from build123d import *

# Parameters (mm, degrees)
SKETCH_1_R          = 22.5
SKETCH_1_R_2        = 1.65
EXTRUDE_1_DEPTH     = 4
SKETCH_2_R          = 12.5
SKETCH_2_R_2        = 8
EXTRUDE_2_DEPTH     = 10
SKETCH_3_R          = 4
CUT_EXTRUDE_1_DEPTH = 3
SKETCH_4_R          = 8
EXTRUDE_3_DEPTH     = 2
SKETCH_3_3_R        = 1.6
CUT_EXTRUDE_2_DEPTH = 10
CHAMFER_1_SIZE      = 2
CHAMFER_1_SIZE2     = 3.464101615


with BuildPart() as part:
    # Sketch 1 → Extrude 1 (new body)
    with BuildSketch(Plane(origin=(0, 0, 0), x_dir=(1, 0, 0), z_dir=(0, 1, 0))):
        with Locations(Location((0, 0, 0), (0, 0, 270))):
            Circle(SKETCH_1_R)
        with Locations(Location((-18, 0, 0), (0, 0, 270))):
            Circle(SKETCH_1_R_2, mode=Mode.SUBTRACT)
        with Locations(Location((18, 0, 0), (0, 0, 270))):
            Circle(SKETCH_1_R_2, mode=Mode.SUBTRACT)
        with Locations(Location((0, 18, 0), (0, 0, 270))):
            Circle(SKETCH_1_R_2, mode=Mode.SUBTRACT)
        with Locations(Location((0, -18, 0), (0, 0, 270))):
            Circle(SKETCH_1_R_2, mode=Mode.SUBTRACT)
    extrude(amount=EXTRUDE_1_DEPTH)

    # Sketch 2 → Extrude 2 (add)
    with BuildSketch(Plane(origin=(0, 4, 0), x_dir=(1, 0, 0), z_dir=(0, 1, 0))):
        with Locations(Location((0, 0, 0), (0, 0, 270))):
            Circle(SKETCH_2_R)
        with Locations(Location((0, 0, 0), (0, 0, 270))):
            Circle(SKETCH_2_R_2, mode=Mode.SUBTRACT)
    extrude(amount=EXTRUDE_2_DEPTH)

    # Sketch 3 → Cut-Extrude 1 (cut)
    with BuildSketch(Plane.XZ):
        with Locations(Location((0, 0, 0), (0, 0, 270))):
            Circle(SKETCH_3_R)
    extrude(amount=-CUT_EXTRUDE_1_DEPTH, mode=Mode.SUBTRACT)

    # Sketch 4 → Extrude 3 (add)
    with BuildSketch(Plane(origin=(0, 4, 0), x_dir=(1, 0, 0), z_dir=(0, 1, 0))):
        with Locations(Location((0, 0, 0), (0, 0, 270))):
            Circle(SKETCH_4_R)
    extrude(amount=EXTRUDE_3_DEPTH)

    # Sketch 3_3 → Cut-Extrude 2 (cut)
    with BuildSketch(Plane.XZ):
        with Locations(Location((0, 0, 0), (0, 0, 270))):
            Circle(SKETCH_3_3_R)
    extrude(amount=-CUT_EXTRUDE_2_DEPTH, mode=Mode.SUBTRACT)

    # Chamfer 1
    chamfer_1_edges = [part.edges().sort_by_distance(p)[0] for p in [
        (0, 4, -12.5),
    ]]
    chamfer_1_side = [part.faces().sort_by_distance(p)[0] for p in [
        (0, 4, -21.863603897),
    ]]
    chamfer(chamfer_1_edges, length=CHAMFER_1_SIZE, length2=CHAMFER_1_SIZE2, reference=chamfer_1_side[0])


solid = part.part
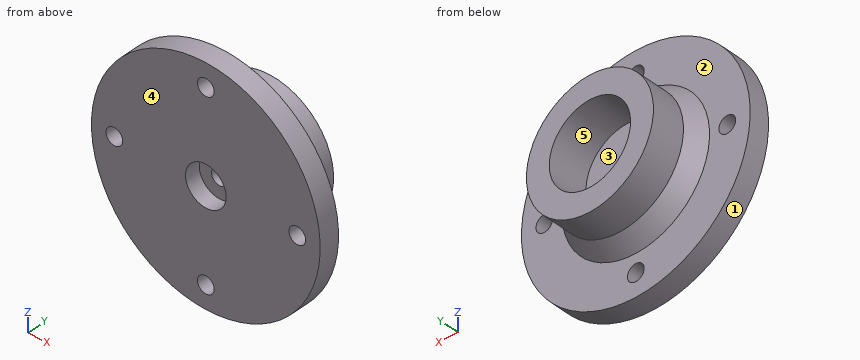
Geometry: final body of the model. Coordinates: model frame, mm. Face numbers are marked on the shaded views. A direction names the side the tool comes from. Round coordinates to 2 decimals unless told otherwise and drop trailing zeros. Loops run counter-clockwise (first coordinate to the right, second up) from the corner with the lowest first, then second, coordinate; pieces in that order, holes last. Notation, with made-up numbers: (84.5, -35) - (100.5, -35) arc R22 cw to (100.5, 4) - close; hole circle Ø9 at (4, 14.25). An arc over 180 degrees is marked (long way). Write each question's results on one line, items separated by ' | '. Start each with the question number.
1) Mould query, pull axis X, two halves, no side actions, for the marked faces 1, 2 and 3. Classes: released by +X, released by -X, zero draft, split by the parting line, or undercut.
2) Access query for the marked faces 4 and 5. Directions: +Z, -Z, +X, -X, +Y, -Y. A direction counts if a zero-diameter tool reaches every point of the face in a straight line with its end or side. Return the directions, or none.
3) Cut plane A-A on x = 18. Return loops of the section in (y, z), then the cut area to 3 significant figures.
4) Line query: probe 1 along X at (y, z) = (0.95, 0); probe 2 along X at (y, z) = (3.05, 0); probe 3 along X at (y, z) = (12, 0). Output: solid intervals per line, ascending. Write a range as [from, to].
5) Cut plane B-B on z = 0. Count the separate pieces of the cut face and the enclosed holes in it, then the cut area to 3 significant figures.
6) Cut plane D-D on z = 18. Return loops of the section in (x, y).
7) First-contact query: P1, Ø5, axis at x = 0, z = 0, coming from the -Y side; P2, Ø5, axis at y = 10.5, z = -10, coming from the +X side; P3, Ø8, axis at y = 6.5, z = 3.5, coming from the +X side. Flat tips, straight axial feed; report the tip coordinate or a pass-through.
Verdict:
1) face 1: split by the parting line | face 2: zero draft | face 3: undercut
2) face 4: +Z, -Z, +X, -X, -Y | face 5: +Y
3) outline: (0, -13.5) - (4, -13.5) - (4, -1.65) - (0, -1.65) - close; (0, 1.65) - (4, 1.65) - (4, 13.5) - (0, 13.5) - close | area: 94.8 mm2
4) probe 1: x = [-22.5, -19.65], [-16.35, -4], [4, 16.35], [19.65, 22.5] | probe 2: x = [-22.5, -19.65], [-16.35, -1.6], [1.6, 16.35], [19.65, 22.5] | probe 3: x = [-12.5, -8], [8, 12.5]
5) separate pieces: 4 | enclosed holes: 0 | area: 249 mm2
6) outline: (-13.5, 0) - (-1.65, 0) - (-1.65, 4) - (-13.5, 4) - close; (1.65, 0) - (13.5, 0) - (13.5, 4) - (1.65, 4) - close
7) P1: stops at y = 3 | P2: stops at x = 10 | P3: stops at x = 22.5
